Part model, mm, in its own coordinate system. A direction names the side the tool comes from. Coordinates: 2 decimals unless noted, no trailing zeros. Write each loop counter-clockwise with the first axis right and the second up, starting at its lowest first coordinate (ties: lowest second). Pieces come first, ordered by that corner, then holes. Notation, with made-up numbers: (82.25, -30) - (114.25, -30) arc R25 cw to (114.25, -15) - close; hole circle Ø8 at (3.5, 29.5). An arc over 180 degrees is marked (long way). Use a Markdown table: item, result.
```python
from build123d import *

# Parameters (mm, degrees)
CROQUIS1_R              = 40
SALIENTE_EXTRUIR1_DEPTH = 2
CROQUIS2_R              = 40
CROQUIS2_R_2            = 35
SALIENTE_EXTRUIR2_DEPTH = 30
CORTAR_EXTRUIR1_START   = -15
CROQUIS3_R              = 37.5
CROQUIS3_R_2            = 35
CORTAR_EXTRUIR1_DEPTH   = 15
CHAFL_N1_SIZE           = 2.5


with BuildPart() as part:
    # Croquis1 → Saliente-Extruir1 (new body)
    with BuildSketch(Plane(origin=(0, 0, 0), x_dir=(1, 0, 0), z_dir=(0, 1, 0))):
        with Locations(Location((0, 0, 0), (0, 0, 270))):
            Circle(CROQUIS1_R)
    extrude(amount=SALIENTE_EXTRUIR1_DEPTH)

    # Croquis2 → Saliente-Extruir2 (add)
    with BuildSketch(Plane(origin=(0, 2, 0), x_dir=(1, 0, 0), z_dir=(0, 1, 0))):
        with Locations(Location((0, 0, 0), (0, 0, 270))):
            Circle(CROQUIS2_R)
        with Locations(Location((0, 0, 0), (0, 0, 270))):
            Circle(CROQUIS2_R_2, mode=Mode.SUBTRACT)
    extrude(amount=SALIENTE_EXTRUIR2_DEPTH)

    # Croquis3 → Cortar-Extruir1 (cut)
    with BuildSketch(Plane(origin=(0, 32, 0), x_dir=(1, 0, 0), z_dir=(0, 1, 0)).offset(CORTAR_EXTRUIR1_START)):
        with Locations(Location((0, 0, 0), (0, 0, 270))):
            Circle(CROQUIS3_R)
        with Locations(Location((0, 0, 0), (0, 0, 270))):
            Circle(CROQUIS3_R_2, mode=Mode.SUBTRACT)
    extrude(amount=CORTAR_EXTRUIR1_DEPTH, mode=Mode.SUBTRACT)

    # Chaflán1
    chafl_n1_edges = [part.edges().sort_by_distance(p)[0] for p in [
        (0, 17, -35),
    ]]
    chamfer(chafl_n1_edges, length=CHAFL_N1_SIZE - 0.0001)  # a hair under: the kernel refuses the full size


solid = part.part
```
Item 1: Two-plate mould, pull along X, no slides. Class faces 3 (the face through (10.55, 14.62, 33.5)), 4 (the face through (1, 0, -1)), 5 (the face through (-39.05, 15.78, -8.67)): pulls with the +X half, pulls with the -X half, needs draft (parallel to the pull), parting line crosses it, or undercut.
From the geometry:
| item | result |
|---|---|
| face 3 | undercut |
| face 4 | needs draft |
| face 5 | parting line crosses it |
Item 2: Which spindle directions (+Z, -Z, +X, -X, +Y, -Y) get a long thin tool onto all of the face, cutting with end or side? Do faces 1 (the face through (-21, 8, -28)), 2 (the face through (36, 32, 12)). Say none if no direction does.
From the geometry:
| item | result |
|---|---|
| face 1 | +Y |
| face 2 | +Z, -Z, +X, -X, +Y |
Item 3: Drill centre lines: probe 1 along X at (y, z) = (20, 0); probe 2 along X at (y, z) = (5, 0); probe 3 along Y at (x, z) = (1, 17.5). Where is each one in solid material? Low to high.
From the geometry:
| item | result |
|---|---|
| probe 1 | -40 to -37.5, 37.5 to 40 |
| probe 2 | -40 to -35, 35 to 40 |
| probe 3 | 0 to 2 |
Item 4: Band-saw the part on B-B, the plane y = 3.5. Give the cut face in (x, z).
From the geometry:
| item | result |
|---|---|
| outline | circle Ø80 at (0, 0); hole circle Ø70 at (0, 0) |
Item 5: Band-saw the part on D-D, the plane y = 18. Give the cut face in (x, z).
From the geometry:
| item | result |
|---|---|
| outline | circle Ø80 at (0, 0); hole circle Ø75 at (0, 0) |
Item 6: Drop flat-ended pins along their axis: P1, Ø2, axis at x = 30, y = 16.5, coming from the +Z side; P2, Ø1.5, axis at x = -11, y = 22.5, coming from the +Z side; P3, Ø6, axis at y = 4, z = -25.5, coming from the +X side. Give the stop position or say it passes through.
From the geometry:
| item | result |
|---|---|
| P1 | z = 27.55 |
| P2 | z = 38.66 |
| P3 | x = 33.07 |
